```python
from build123d import *

# Parameters (mm, degrees)
SALIENTE_EXTRUIR1_DEPTH = 10.1
CROQUIS7_R              = 2.05
CORTAR_EXTRUIR1_DEPTH   = 0.5
CROQUIS11_W             = 20
CROQUIS11_H             = 1.2
CORTAR_EXTRUIR4_DEPTH   = 49.726011614
SALIENTE_EXTRUIR2_START = -7.7
SALIENTE_EXTRUIR2_DEPTH = 7.7
CROQUIS15_R             = 2.5
CORTAR_EXTRUIR5_DEPTH   = 1.5


with BuildPart() as part:
    # Croquis1 → Saliente-Extruir1 (new body)
    with BuildSketch(Plane(origin=(0, 0, 0), x_dir=(1, 0, 0), z_dir=(0, 1, 0))):
        with BuildLine():
            Line((-32.835114186, -4.991653889), (32.944915669, -4.991653889))
            Line((32.944915669, -4.991653889), (32.944915669, 5.008346111))
            Line((32.944915669, 5.008346111), (-33.055084331, 5.008346111))
            ThreePointArc((-33.055084331, 5.008346111), (-46.031021583, -0.279505113), (-32.835114186, -4.991653889))
        make_face()
    extrude(amount=SALIENTE_EXTRUIR1_DEPTH)

    # Croquis7 → Cortar-Extruir1 (cut)
    with BuildSketch(Plane(origin=(0, 10.1, 0), x_dir=(1, 0, 0), z_dir=(0, 1, 0))):
        with Locations(Location((-38.532835433, -0.114567403, 0), (0, 0, 270))):
            Circle(CROQUIS7_R)
    extrude(amount=-CORTAR_EXTRUIR1_DEPTH, mode=Mode.SUBTRACT)

    # Croquis11 → Cortar-Extruir4 (cut, through all)
    with BuildSketch(Plane.XY.offset(4.991653889)):
        with Locations((22.944915669, 9.5)):
            Rectangle(CROQUIS11_W, CROQUIS11_H)
        with Locations((22.944915669, 0.6)):
            Rectangle(CROQUIS11_W, CROQUIS11_H)
    extrude(amount=-CORTAR_EXTRUIR4_DEPTH, mode=Mode.SUBTRACT)

    # Croquis14 → Saliente-Extruir2 (add)
    with BuildSketch(Plane(origin=(0, 8.9, 0), x_dir=(1, 0, 0), z_dir=(0, 1, 0)).offset(SALIENTE_EXTRUIR2_START)):
        with BuildLine():
            Line((32.944915669, 5.008346111), (32.944915669, -4.991653889))
            ThreePointArc((32.944915669, -4.991653889), (38.512321796, -4.082434131), (43.501214134, -1.449252634))
            ThreePointArc((43.501214134, -1.449252634), (44.473014214, 5.554717998), (37.469043582, 6.526518077))
            ThreePointArc((37.469043582, 6.526518077), (35.330946866, 5.398011722), (32.944915669, 5.008346111))
        make_face()
    extrude(amount=SALIENTE_EXTRUIR2_DEPTH)

    # Croquis15 → Cortar-Extruir5 (cut)
    with BuildSketch(Plane(origin=(0, 8.9, 0), x_dir=(1, 0, 0), z_dir=(0, 1, 0))):
        with Locations(Location((40.485128858, 2.538632722, 0), (0, 0, 270))):
            Circle(CROQUIS15_R)
    cortar_extruir5 = extrude(amount=-CORTAR_EXTRUIR5_DEPTH, mode=Mode.SUBTRACT)

    # Simetría1: Cortar-Extruir5 across plane
    add(cortar_extruir5.mirror(Plane.ZX.offset(5.05)), mode=Mode.SUBTRACT)


solid = part.part
```
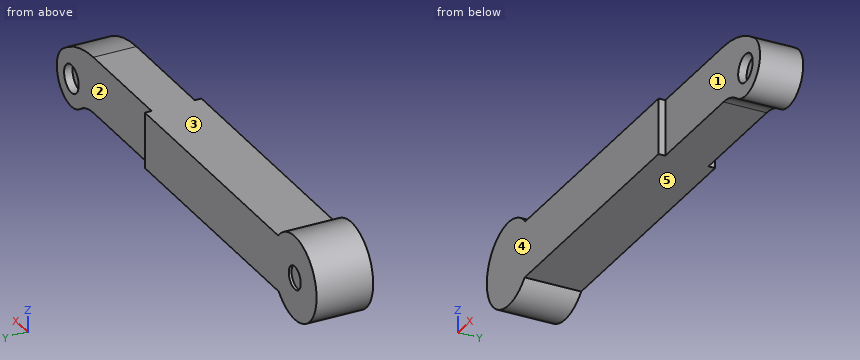
Can you work these out from the model? Positions are in its coordinate system, mm. Face numbers are marked on the shaded views. A direction names the side the tool comes from. Round coordinates to 2 decimals unless told otherwise and drop trailing zeros. Order: outer loops, then holes, each group sorted by start corner. A loop starts at its lowest first (then second) coordinate and runs counter-clockwise, first axis right, second up.
(1) If we section it at B-B (z = -3.5): Please give me the cut outline in (x, y), plus the area to 3 significant figures.
Results are:
outline: (-45.1, 0) - (12.94, 0) - (12.94, 1.2) - (38.18, 1.2) - (38.18, 2.7) - (42.79, 2.7) - (42.79, 1.2) - (45.39, 1.2) - (45.39, 8.9) - (42.79, 8.9) - (42.79, 7.4) - (38.18, 7.4) - (38.18, 8.9) - (12.94, 8.9) - (12.94, 10.1) - (-45.1, 10.1) - close
area: 822 mm2
(2) I'm going to push flat-ended pins straight in: pin 1 (3 mm diameter, centred on y = 2.5, z = 3.5, fed in from +X); pin 2 (4 mm diameter, centred on x = 24.5, z = 2, fed in from +Y); pin 3 (2.5 mm diameter, centred on x = 41.5, z = -2.5, fed in from -Y); pin 4 (1.5 mm diameter, centred on x = -30, z = 2, fed in from -Y). Where does each tip first touch, or does it pass through?
Results are:
pin 1: stops at x = 42.73
pin 2: stops at y = 8.9
pin 3: stops at y = 2.7
pin 4: stops at y = 0
(3) If I drill on L1, parallel to Z at x = 10.5, y = 4; L2, parallel to Y at x = 17.5, z = 4.75; L3, parallel to X at y = 1.5, z = 0.5, over which ranges is the centre line in solid material (lowest first)?
Results are:
L1: z = -5.01 to 4.99
L2: y = 1.2 to 8.9
L3: x = -46.02 to 44.46
(4) If we section it at C-C (x = -18): Please give me the cut outline in (y, z).
Results are:
outline: (0, -5.01) - (10.1, -5.01) - (10.1, 4.99) - (0, 4.99) - close
(5) On a 3-axis mill with a long thin cutter (end or side, diameter ignored), from which of +Z, -Z, +X, -X, +Y, -Y can I reach the whole of each face in a straight line? I mean the marked faces 1, 2 and 3. Say none if no direction works.
Results are:
face 1: +Z, -Z, +X, -Y
face 2: +Z, -Z, +X, +Y
face 3: +Z, +X, +Y, -Y
(6) If we section it at D-D (x = 20): Please give me the cut outline in (y, z).
Results are:
outline: (1.2, -5.01) - (8.9, -5.01) - (8.9, 4.99) - (1.2, 4.99) - close
(7) We'd pull the mould along X, two halves only. Please class the marked faces 4 and 5: +X half, -X half, draft (parallel to the pull), parting line (faces both ways), or undercut.
Results are:
face 4: draft
face 5: undercut
(8) If we section it at A-A (y = 5.5): Please give me the cut outline in (x, z), plus the area to 3 significant figures.
Results are:
outline: (-33.06, -5.01) - (32.94, -5.01) arc R7.5 cw to (37.47, -6.53) arc R5 ccw to (43.5, 1.45) arc R17.5 ccw to (32.94, 4.99) - (-32.84, 4.99) arc R7.5 ccw (long way) to start
area: 943 mm2
